Drawing for the job (mm, zero at the part's lowest x, y, z). A direction names the side the tool comes from. Give positions to 0.01 mm unless a question says otherwise; leave off trailing zeros. Order: outer loops, then holes, each group sorted by start corner. A loop starts at its lowest first (then second) coordinate and runs counter-clockwise, first axis right, second up. Notation, with made-up numbers: (37.25, 21) - (96.25, 21) arc R18 cw to (96.25, 43) - close; hole circle Ø4 at (69, 88). An arc over 180 degrees is marked (long way). One line per item, written item: value.
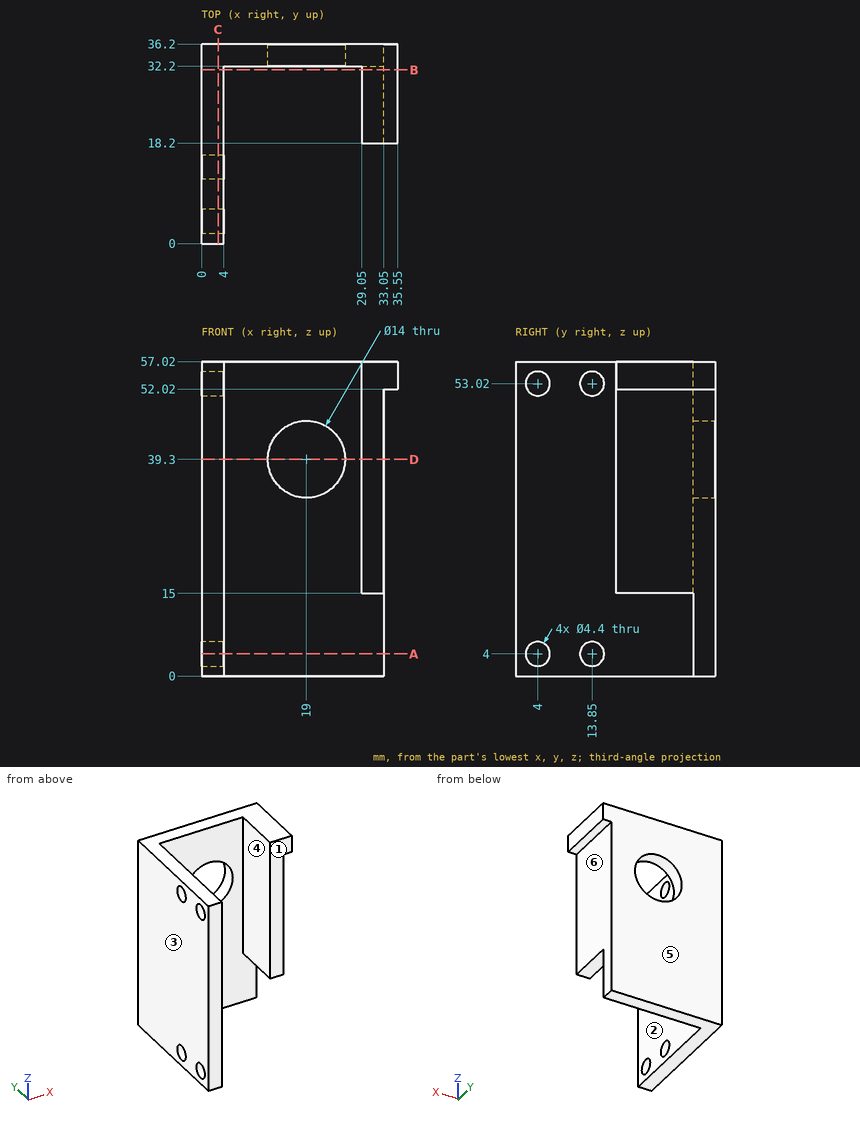
(1) Slice it at A-A, the plane z = 4. Give the cut face in (x, y), and give its area (3 significant figures).
Completed:
outline: (0, 0) - (4, 0) - (4, 1.8) - (0, 1.8) - close; (0, 6.2) - (4, 6.2) - (4, 11.65) - (0, 11.65) - close; (0, 16.05) - (4, 16.05) - (4, 32.2) - (33.05, 32.2) - (33.05, 36.2) - (0, 36.2) - close
area: 226 mm²
(2) Slice it at D-D, the plane z = 39.3. Give the cut face in (x, y).
Completed:
outline: (0, 0) - (4, 0) - (4, 32.2) - (12, 32.2) - (12, 36.2) - (0, 36.2) - close; (26, 32.2) - (29.05, 32.2) - (29.05, 18.2) - (33.05, 18.2) - (33.05, 36.2) - (26, 36.2) - close
(3) Drill centre lines: line 1 (Y direction, x = 2.1, z = 53.02); line 2 (X direction, y = 28, z = 29); line 3 (X direction, y = 33, z = 39). Where is each one in solid material? Low to high.
Completed:
line 1: 0 to 1.8, 6.2 to 11.65, 16.05 to 36.2
line 2: 0 to 4, 29.05 to 33.05
line 3: 0 to 12.01, 25.99 to 33.05
(4) 3-axis set-ups, long thin cutter, end or side, ignore diameter. For the marked faces 4, 5 and 6: which of +Z, -Z, +X, -X, +Y, -Y reach the whole face in a straight line?
Completed:
face 4: +Z, -Z, -Y
face 5: +Z, -Z, +X, -X, +Y
face 6: -Z, +X, +Y, -Y
(5) Pull direction X, two halves, no side cores. Call the marked faces 1, 2 and 3: +X half, -X half, draft (parallel to the pull), parting line (faces both ways), or undercut.
Completed:
face 1: draft
face 2: undercut
face 3: -X half
(6) Slice it at C-C, the plane x = 3. Give the cut face in (y, z).
Completed:
outline: (0, 0) - (36.2, 0) - (36.2, 57.02) - (0, 57.02) - close; hole circle Ø4.4 at (4, 4); hole circle Ø4.4 at (4, 53.02); hole circle Ø4.4 at (13.85, 4); hole circle Ø4.4 at (13.85, 53.02)
(7) Slice it at B-B, the plane y = 31.5. Give the cut face in (x, z).
Completed:
outline: (0, 0) - (4, 0) - (4, 57.02) - (0, 57.02) - close; (29.05, 15) - (33.05, 15) - (33.05, 52.02) - (35.55, 52.02) - (35.55, 57.02) - (29.05, 57.02) - close
(8) Pin check, flat tips, straight feed: P1, Ø5, axis at y = 13.85, z = 4, coming from the +X side; P2, Ø2, axis at y = 32.5, z = 36, coming from the +X side; P3, Ø1.2, axis at x = 34.5, y = 25.5, coming from the -Z side. Stop position of each tip, or through.
Completed:
P1: x = 4
P2: x = 33.05
P3: z = 52.02
